Source: CAD feature listing. Evaluate the final solid. Frame: model axes, mm. A direction names the side the tool comes from. Coordinates: 2 decimals unless noted, no trailing zeros. Order: outer loops, then holes, each group sorted by start corner. A loop starts at its lowest first (then second) coordinate and runs counter-clockwise, first axis right, second up.
```python
from build123d import *

# Parameters (mm, degrees)
SKETCH1_W           = 38.1
SKETCH1_H           = 38.1
BOSS_EXTRUDE1_DEPTH = 7.62
SKETCH2_R           = 18
SKETCH2_R_2         = 6.35
BOSS_EXTRUDE2_DEPTH = 1.27
SKETCH5_R           = 6.35
CUT_EXTRUDE1_DEPTH  = 31.365983763
SKETCH4_R           = 2.54
CUT_EXTRUDE2_DEPTH  = 7.62
CUT_EXTRUDE3_START  = -7.62
SKETCH6_R           = 2.54
CUT_EXTRUDE3_DEPTH  = 7.62


with BuildPart() as part:
    # Sketch1 → Boss-Extrude1 (new body)
    with BuildSketch(Plane(origin=(0, 0, 0), x_dir=(1, 0, 0), z_dir=(0, 1, 0))):
        with Locations((-0.926041667, 2.513541667)):
            Rectangle(SKETCH1_W, SKETCH1_H)
    extrude(amount=BOSS_EXTRUDE1_DEPTH)

    # Sketch2 → Boss-Extrude2 (add)
    with BuildSketch(Plane(origin=(0, 7.62, 0), x_dir=(1, 0, 0), z_dir=(0, 1, 0))):
        with Locations(Location((-0.926041667, 2.513541667, 0), (0, 0, 270))):
            Circle(SKETCH2_R)
        with Locations(Location((-0.926041667, 2.513541667, 0), (0, 0, 270))):
            Circle(SKETCH2_R_2, mode=Mode.SUBTRACT)
    extrude(amount=BOSS_EXTRUDE2_DEPTH)

    # Sketch5 → Cut-Extrude1 (cut, through all)
    with BuildSketch(Plane(origin=(0, 7.62, 0), x_dir=(1, 0, 0), z_dir=(0, 1, 0))):
        with Locations(Location((-0.926041667, 2.513541667, 0), (0, 0, 270))):
            Circle(SKETCH5_R)
    extrude(amount=-CUT_EXTRUDE1_DEPTH, mode=Mode.SUBTRACT)

    # Sketch4 → Cut-Extrude2 (cut)
    with BuildSketch(Plane.ZY.offset(19.976041667)):
        with Locations((-12.038541667, 3.81)):
            Circle(SKETCH4_R)
        with Locations((7.011458333, 3.81)):
            Circle(SKETCH4_R)
    extrude(amount=-CUT_EXTRUDE2_DEPTH, mode=Mode.SUBTRACT)

    # Sketch6 → Cut-Extrude3 (cut)
    with BuildSketch(Plane(origin=(18.123958333, 0, 0), x_dir=(0, 0, -1), z_dir=(1, 0, 0)).offset(CUT_EXTRUDE3_START)):
        with Locations(Location((-7.011458333, 3.81, 0), (0, 0, 180))):
            Circle(SKETCH6_R)
        with Locations(Location((12.038541667, 3.81, 0), (0, 0, 180))):
            Circle(SKETCH6_R)
    extrude(amount=CUT_EXTRUDE3_DEPTH, mode=Mode.SUBTRACT)


solid = part.part
```
1. Contact query for flat-ended pins moving along their axis: P1, Ø4, axis at y = 3.81, z = -12.04, coming from the +X side; P2, Ø2.5, axis at y = 4.5, z = -11.5, coming from the -X side; P3, Ø14.5, axis at x = -0.93, z = -2.51, coming from the -Y side. Output: stop coordinate, or through.
2. Draft query along Y for faces 1 (the flat face through (-1, 0, -11)), 2 (the flat face through (-12.356, 4, -12)), 3 (the flat face through (-8, 7.62, -20)), 4 (the flat face through (-1, 4, -21.564)). Return one class per face: +Y half, -Y half, draft (parallel to the pull), parting line (faces both ways), or undercut.
3. Material intervals for line 1 along Z through (x, y) = (12.5, 3.75); line 2 along X through (y, z) = (1.25, -2.5); line 3 along Z through (x, y) = (-17.5, 5), sorted ascending.
4. Section query D-D, the plane x = 16. Output: boundary loops of the cut face in (y, z), plus the area to 3 significant figures.
5. Section query B-B, the plane x = 2. Output: boundary loops of the cut face in (y, z).
6. Section query A-A, the plane z = 0. Output: boundary loops of the cut face in (x, y), plus the area to 3 significant figures.
7. Access query for faces 5 (the flat face through (-1, 4, 16.536)), 6 (the cylindrical face through (4.481, 8.246, 14.655)), 7 (the flat face through (18.124, 4, -2)), 8 (the flat face through (-12.356, 4, 7)), 9 (the flat face through (10.504, 4, 7)). Directions: +Z, -Z, +X, -X, +Y, -Y. A direction counts if a zero-diameter tool reaches every point of the face in a straight line with its end or side. Return the directions, or none.
8. Section query C-C, the plane y = 3.25. Output: boundary loops of the cut face in (x, z), plus the area to 3 significant figures.
Answer key:
1. P1: stops at x = 10.5
1. P2: stops at x = -12.36
1. P3: stops at y = 0
2. face 1: -Y half
2. face 2: undercut
2. face 3: +Y half
2. face 4: draft
3. line 1: z = -21.56 to -14.58, -9.5 to 4.47, 9.55 to 16.54
3. line 2: x = -19.98 to -7.28, 5.42 to 18.12
3. line 3: z = -21.56 to -14.28, -9.79 to 4.77, 9.26 to 16.54
4. outline: (0, -21.56) - (7.62, -21.56) - (7.62, -8.64) - (8.89, -8.64) - (8.89, 3.61) - (7.62, 3.61) - (7.62, 16.54) - (0, 16.54) - close; hole circle Ø5.08 at (3.81, -12.04); hole circle Ø5.08 at (3.81, 7.01)
4. area: 265 mm2
5. outline: (0, -21.56) - (7.62, -21.56) - (7.62, -20.27) - (8.89, -20.27) - (8.89, -8.15) - (0, -8.15) - close; (0, 3.12) - (8.89, 3.12) - (8.89, 15.25) - (7.62, 15.25) - (7.62, 16.54) - (0, 16.54) - close
6. outline: (-19.98, 0) - (-6.76, 0) - (-6.76, 8.89) - (-18.75, 8.89) - (-18.75, 7.62) - (-19.98, 7.62) - close; (4.91, 0) - (18.12, 0) - (18.12, 7.62) - (16.9, 7.62) - (16.9, 8.89) - (4.91, 8.89) - close
6. area: 232 mm2
7. face 5: +Z, +X, -X, +Y, -Y
7. face 6: +Y
7. face 7: +Z, -Z, +X, +Y, -Y
7. face 8: -X
7. face 9: +X
8. outline: (-19.98, -21.56) - (18.12, -21.56) - (18.12, -14.52) - (10.5, -14.52) - (10.5, -9.56) - (18.12, -9.56) - (18.12, 4.53) - (10.5, 4.53) - (10.5, 9.49) - (18.12, 9.49) - (18.12, 16.54) - (-19.98, 16.54) - (-19.98, 9.49) - (-12.36, 9.49) - (-12.36, 4.53) - (-19.98, 4.53) - (-19.98, -9.56) - (-12.36, -9.56) - (-12.36, -14.52) - (-19.98, -14.52) - close; hole circle Ø12.7 at (-0.93, -2.51)
8. area: 1,170 mm2
